Geometry check sheet. Reference: the model listing, model coordinates, mm. A direction names the side the tool comes from. Give positions to 0.01 mm unless a question says otherwise; leave off trailing zeros. Order: outer loops, then holes, each group sorted by start corner. A loop starts at its lowest first (then second) coordinate and runs counter-clockwise, first axis right, second up. Notation, with made-up numbers: M 8,48 L 52,48 A21 cw 52,59 Z; hole C 73,27.25 d1. An arc over 180 degrees is marked long. Answer as CSV lines item,"result".
from build123d import *

# Parameters (mm, degrees)
SKETCH1_R           = 8.5
BOSS_EXTRUDE1_DEPTH = 4.4
SKETCH3_R           = 5.8
CUT_EXTRUDE1_DEPTH  = 4
BOSS_EXTRUDE3_START = 3
SKETCH4_R           = 8.5
SKETCH4_R_2         = 7.5
BOSS_EXTRUDE3_DEPTH = 3
BOSS_EXTRUDE4_DEPTH = 0.6


with BuildPart() as part:
    # Sketch1 → Boss-Extrude1 (new body)
    with BuildSketch(Plane.XY):
        Circle(SKETCH1_R)
    extrude(amount=BOSS_EXTRUDE1_DEPTH)

    # Sketch3 → Cut-Extrude1 (cut)
    with BuildSketch(Plane(origin=(0, 0, 0), x_dir=(-1, 0, 0), z_dir=(0, 0, -1))):
        Circle(SKETCH3_R)
    extrude(amount=-CUT_EXTRUDE1_DEPTH, mode=Mode.SUBTRACT)

    # Sketch4 → Boss-Extrude3 (add)
    with BuildSketch(Plane(origin=(0, 0, 0), x_dir=(-1, 0, 0), z_dir=(0, 0, -1)).offset(BOSS_EXTRUDE3_START)):
        Circle(SKETCH4_R)
        Circle(SKETCH4_R_2, mode=Mode.SUBTRACT)
    extrude(amount=-BOSS_EXTRUDE3_DEPTH)

    # Sketch6 → Cut-Revolve1 (revolve, cut)
    with BuildSketch(Plane(origin=(0, 0, 0), x_dir=(1, 0, 0), z_dir=(0, 1, 0)), mode=Mode.PRIVATE) as cut_revolve1_sk:
        Polygon((7.5, 0), (5.8, -1.7), (5.8, 0), align=None)
    revolve(cut_revolve1_sk.sketch.rotate(Axis((0, 0, -5.5), (0, 0, 1)), 180), axis=Axis((0, 0, -5.5), (0, 0, 1)), mode=Mode.SUBTRACT)

    # Sketch2 → Boss-Extrude4 (add)
    with BuildSketch(Plane.XY.offset(4.4)):
        Polygon((0.086062041, -5.591622222), (-6.919546933, 1.481294445), (-5.949194369, 2.462864958), (0.086062041, -3.628481196), (6.11290499, 2.462864958), (7.080453067, 1.481294445), align=None)
    extrude(amount=BOSS_EXTRUDE4_DEPTH)


solid = part.part
(1) Draft check along X on faces 1 (the face through (6.59, 1.98, 4.7)), 2 (the face through (-1, -3, 5)), 3 (the face through (0, 0, 4.4)). Enter one of: +X half, -X half, draft (parallel to the pull), parting line (faces both ways), or undercut.
The answers:
face 1,"+X half"
face 2,"draft"
face 3,"undercut"
(2) Section check A-A on z = -1.25. Enter the section's corners in (x, y).
The answers:
outline,"C 0,0 d17; hole C 0,0 d15"
(3) Section check D-D on y = 7.75. Enter the section's corners in (x, z), then the cut area to 3 significant figures.
The answers:
outline,"M -3.49,-3 L 3.49,-3 L 3.49,4.4 L -3.49,4.4 Z"
area,"51.7 mm2"
(4) Section check B-B on y = 0. Enter the section's corners in (x, z).
The answers:
outline,"M -8.5,-3 L -7.5,-3 L -7.5,0 L -5.8,1.7 L -5.8,4 L 5.8,4 L 5.8,1.7 L 7.5,0 L 7.5,-3 L 8.5,-3 L 8.5,4.4 L 5.62,4.4 L 5.62,5 L 3.68,5 L 3.68,4.4 L -3.51,4.4 L -3.51,5 L -5.45,5 L -5.45,4.4 L -8.5,4.4 Z"
(5) Section check C-C on z = 2.75. Enter the section's corners in (x, y).
The answers:
outline,"C 0,0 d17; hole C 0,0 d11.6"
(6) Gauge pin test, flat ends, axial feed: P1, Ø4, axis at y = -5, z = 0, coming from the +X side; P2, Ø1, axis at x = 2, z = 0.5, coming from the +Y side; P3, Ø4, axis at x = -3.5, z = 0, coming from the -Y side; P4, Ø8.5, axis at x = 3.5, y = 4, coming from the +Z side. Record the tip position at first contact, or that the pin passes through.
The answers:
P1,"stops at x = 7.95"
P2,"stops at y = 8.37"
P3,"stops at y = -8.37"
P4,"stops at z = 5"
(7) Tool access check on faces 4 (the face through (0, 0, 4)), 5 (the face through (3.63, -2.01, 4.7)), 6 (the face through (3.057, -0.625, 4.696)), 7 (the face through (-3.37, -2.1, 4.7)), 8 (the face through (-6.441, 1.965, 4.696)). Record the directions out of +Z, -Z, +X, -X, +Y, -Y that give a thin tool (end or side, any length) a straight path to the whole face; none if there is none.
The answers:
face 4,"-Z"
face 5,"+Z, +X, -Y"
face 6,"+Z, +Y"
face 7,"+Z, -X, -Y"
face 8,"+Z, -X, +Y"
(8) Material ranges on line 1 (Y direction, x = 0, z = -1.35); line 2 (X direction, y = 0, z = 2.5), recorded low to high.
The answers:
line 1,"y = -8.5 to -7.5, 7.5 to 8.5"
line 2,"x = -8.5 to -5.8, 5.8 to 8.5"
